```python
from build123d import *

# Parameters (mm, degrees)
F1_DEPTH       = 2.54
F3_D           = 4.4
F3_DEPTH       = 37.1856
F3_CSINK_D     = 8.96
F3_CSINK_ANGLE = 90
F3_TIP         = 1.3218933619
F4_W           = 26.1344808769
F4_H           = 86.36
F5_DEPTH       = 1.27
F7_DEPTH       = 25.4


with BuildPart() as f1:
    # F0 (on Right) → F1 (new body)
    with BuildSketch(Plane.YZ):
        Polygon((62.865, 0), (-62.865, 0), (-60.325, -86.36), (60.325, -86.36), align=None)
        Polygon((-60.325, -86.36), (-62.865, 0), (-62.865, -86.36), align=None)
        Polygon((62.865, -86.36), (62.865, 0), (60.325, -86.36), align=None)
    extrude(amount=F1_DEPTH)

    # F3
    with Locations(Plane(origin=(0, 0, 0), x_dir=(0, -1, 0), z_dir=(-1, 0, 0))):
        with Locations((-59.055, -5.08), (0, -5.08), (59.055, -5.08)):
            CounterSinkHole(F3_D / 2, F3_CSINK_D / 2, depth=F3_DEPTH, counter_sink_angle=F3_CSINK_ANGLE)
            with Locations((0, 0, -(F3_DEPTH + F3_TIP / 2))):  # 118° drill point
                Cone(0, F3_D / 2, F3_TIP, mode=Mode.SUBTRACT)

    # F4 (on face) → F5 (cut)
    with BuildSketch(Plane(origin=(0, 0, 0), x_dir=(0, -1, 0), z_dir=(-1, 0, 0))):
        with Locations((-65.7722404385, -43.18)):
            Rectangle(F4_W, F4_H)
        with Locations((65.7722404385, -43.18)):
            Rectangle(F4_W, F4_H)
    extrude(amount=-F5_DEPTH, mode=Mode.SUBTRACT)

    # F6 (on face) → F7 (cut)
    with BuildSketch(Plane(origin=(0, 0, 0), x_dir=(0, -1, 0), z_dir=(-1, 0, 0))):
        Polygon((0, -80.01), (-38.1, -86.36), (38.1, -86.36), align=None)
        Polygon((-40.64, -16.929261314), (-46.99, -16.929261314), (-50.165, -22.4285226281), (-46.99, -27.9277839421), (-40.64, -27.9277839421), (-37.465, -22.4285226281), align=None)
        Polygon((-40.64, -30.4677839421), (-46.99, -30.4677839421), (-50.165, -35.9670452561), (-46.99, -41.4663065701), (-40.64, -41.4663065701), (-37.465, -35.9670452561), align=None)
        Polygon((-40.64, -44.0063065701), (-46.99, -44.0063065701), (-50.165, -49.5055678841), (-46.99, -55.0048291981), (-40.64, -55.0048291981), (-39.0525, -52.2551985411), (-37.465, -49.5055678841), align=None)
        Polygon((-34.925, -37.2370452561), (-38.1, -42.7363065701), (-34.925, -48.2355678841), (-28.575, -48.2355678841), (-25.4, -42.7363065701), (-28.575, -37.2370452561), align=None)
        Polygon((-34.925, -34.6970452561), (-28.575, -34.6970452561), (-25.4, -29.1977839421), (-28.575, -23.698522628), (-34.925, -23.698522628), (-38.1, -29.1977839421), align=None)
        Polygon((-34.925, -21.1585226281), (-28.575, -21.1585226281), (-25.4, -15.659261314), (-28.575, -10.16), (-34.925, -10.16), (-38.1, -15.659261314), align=None)
        Polygon((-28.575, -50.7755678841), (-34.925, -50.7755678841), (-38.1, -56.2748291981), (-34.925, -61.7740905122), (-28.575, -61.7740905122), (-25.4, -56.2748291981), align=None)
        Polygon((-12.7, -29.1977839421), (-9.525, -34.6970452561), (-3.175, -34.6970452561), (0, -29.1977839421), (-3.175, -23.698522628), (-9.525, -23.698522628), align=None)
        Polygon((-12.065, -35.9670452561), (-15.24, -30.4677839421), (-21.59, -30.4677839421), (-24.765, -35.9670452561), (-21.59, -41.4663065701), (-15.24, -41.4663065701), align=None)
        Polygon((-3.175, -61.7740905122), (0, -56.2748291981), (-3.175, -50.7755678841), (-9.525, -50.7755678841), (-12.7, -56.2748291981), (-9.525, -61.7740905122), align=None)
        Polygon((-9.525, -10.16), (-12.7, -15.659261314), (-9.525, -21.1585226281), (-3.175, -21.1585226281), (0, -15.659261314), (-3.175, -10.16), align=None)
        Polygon((-12.065, -49.5055678841), (-15.24, -44.0063065701), (-21.59, -44.0063065701), (-24.765, -49.5055678841), (-21.59, -55.0048291981), (-15.24, -55.0048291981), (-13.6525, -52.2551985411), align=None)
        Polygon((-15.24, -27.9277839421), (-12.065, -22.4285226281), (-15.24, -16.929261314), (-21.59, -16.929261314), (-24.765, -22.4285226281), (-21.59, -27.9277839421), align=None)
        Polygon((-12.7, -42.7363065701), (-9.525, -48.2355678841), (-3.175, -48.2355678841), (0, -42.7363065701), (-3.175, -37.2370452561), (-9.525, -37.2370452561), align=None)
        Polygon((12.7, -29.1977839421), (15.875, -34.6970452561), (22.225, -34.6970452561), (25.4, -29.1977839421), (22.225, -23.698522628), (15.875, -23.698522628), align=None)
        Polygon((13.335, -35.9670452561), (10.16, -30.4677839421), (3.81, -30.4677839421), (0.635, -35.9670452561), (3.81, -41.4663065701), (10.16, -41.4663065701), align=None)
        Polygon((22.225, -61.7740905122), (25.4, -56.2748291981), (22.225, -50.7755678841), (15.875, -50.7755678841), (12.7, -56.2748291981), (15.875, -61.7740905122), align=None)
        Polygon((15.875, -10.16), (12.7, -15.659261314), (15.875, -21.1585226281), (22.225, -21.1585226281), (25.4, -15.659261314), (22.225, -10.16), align=None)
        Polygon((13.335, -49.5055678841), (10.16, -44.0063065701), (3.81, -44.0063065701), (0.635, -49.5055678841), (3.81, -55.0048291981), (10.16, -55.0048291981), (11.7475, -52.2551985411), align=None)
        Polygon((10.16, -27.9277839421), (13.335, -22.4285226281), (10.16, -16.929261314), (3.81, -16.929261314), (0.635, -22.4285226281), (3.81, -27.9277839421), align=None)
        Polygon((12.7, -42.7363065701), (15.875, -48.2355678841), (22.225, -48.2355678841), (25.4, -42.7363065701), (22.225, -37.2370452561), (15.875, -37.2370452561), align=None)
        Polygon((38.1, -29.1977839421), (41.275, -34.6970452561), (47.625, -34.6970452561), (50.8, -29.1977839421), (47.625, -23.698522628), (41.275, -23.698522628), align=None)
        Polygon((38.735, -35.9670452561), (35.56, -30.4677839421), (29.21, -30.4677839421), (26.035, -35.9670452561), (29.21, -41.4663065701), (35.56, -41.4663065701), align=None)
        Polygon((47.625, -61.7740905122), (50.8, -56.2748291981), (47.625, -50.7755678841), (41.275, -50.7755678841), (38.1, -56.2748291981), (41.275, -61.7740905122), align=None)
        Polygon((41.275, -10.16), (38.1, -15.659261314), (41.275, -21.1585226281), (47.625, -21.1585226281), (50.8, -15.659261314), (47.625, -10.16), align=None)
        Polygon((38.735, -49.5055678841), (35.56, -44.0063065701), (29.21, -44.0063065701), (26.035, -49.5055678841), (29.21, -55.0048291981), (35.56, -55.0048291981), (37.1475, -52.2551985411), align=None)
        Polygon((35.56, -27.9277839421), (38.735, -22.4285226281), (35.56, -16.929261314), (29.21, -16.929261314), (26.035, -22.4285226281), (29.21, -27.9277839421), align=None)
        Polygon((38.1, -42.7363065701), (41.275, -48.2355678841), (47.625, -48.2355678841), (50.8, -42.7363065701), (47.625, -37.2370452561), (41.275, -37.2370452561), align=None)
    extrude(amount=-F7_DEPTH, mode=Mode.SUBTRACT)


solid = f1.part
```
The listing builds one solid part. Answer for the finished solid, in the listing's coordinates (mm). A direction names the side the tool comes from. Coordinates: 2 decimals unless noted, no trailing zeros. Write each loop counter-clockwise with the first axis right and the second up, starting at its lowest first coordinate (ties: lowest second). Pieces come first, ordered by that corner, then holes. Notation, with made-up numbers: (-28, 52) - (27, 52) arc R24 ccw to (27, 64) - close; hole circle Ø4 at (87.5, 76). An arc over 180 degrees is marked (long way). One line per item, written item: value.
1) Find section A-A (z = -5.08). Give the vertices of the cut face in (x, y) (3 decimals).
Geometry check:
outline: (0, -52.705) - (1.27, -52.705) - (1.27, -55.845) - (2.28, -56.855) - (2.54, -56.855) - (2.54, -2.2) - (2.28, -2.2) - (0, -4.48) - close; (0, 4.48) - (2.28, 2.2) - (2.54, 2.2) - (2.54, 56.855) - (2.28, 56.855) - (1.27, 55.845) - (1.27, 52.705) - (0, 52.705) - close; (1.27, -62.865) - (2.54, -62.865) - (2.54, -61.255) - (2.28, -61.255) - (1.27, -62.265) - close; (1.27, 62.265) - (2.28, 61.255) - (2.54, 61.255) - (2.54, 62.865) - (1.27, 62.865) - close
2) Consider line 1 along Y through (x, z) = (2.5, -5.08) (3 decimals); line 2 along Z through (x, y) = (1.85, -42); line 3 along Y through (x, z) = (2.1, -28) (3 decimals). Determine where each line is inside the solid, lowest interval first. Write a range as from..to.
Geometry check:
line 1: y = -62.865..-61.255, -56.855..-2.2, 2.2..56.855, 61.255..62.865
line 2: z = -86.36..-61.77, -50.78..-48.24, -37.24..-34.7, -23.7..-21.16, -10.16..0
line 3: y = -62.865..-50.108, -38.792..-24.708, -13.392..0.692, 12.008..26.092, 37.408..62.865
3) Find section D-D (x = 0.5). Count the separate pieces of the cut face and the enclosed holes in it, and give its area (3 significant figures).
Geometry check:
separate pieces: 1
enclosed holes: 29
area: 5,880 mm2
4) A tool of negligible diameter and unlimited length cuts with its end or side. For faces 1 (the flat face through (1.25, -19.32, -83.23)), 2 (the flat face through (1, -32, -41.466)), 3 (the conical face through (2.169, -0.501, -7.336)), from which of +Z, -Z, +X, -X, +Y, -Y can it reach the whole face along a straight path? Write none if from no direction.
Geometry check:
face 1: -Z, +X, -X
face 2: +X, -X
face 3: -X
5) Find section C-C (z = -59.5). Give the vertices of the cut face in (x, y) (3 decimals).
Geometry check:
outline: (0, -52.705) - (1.27, -52.705) - (1.27, -62.865) - (2.54, -62.865) - (2.54, -48.938) - (0, -48.938) - close; (0, -39.962) - (2.54, -39.962) - (2.54, -23.538) - (0, -23.538) - close; (0, -14.562) - (2.54, -14.562) - (2.54, 1.862) - (0, 1.862) - close; (0, 10.838) - (2.54, 10.838) - (2.54, 27.262) - (0, 27.262) - close; (0, 36.238) - (2.54, 36.238) - (2.54, 62.865) - (1.27, 62.865) - (1.27, 52.705) - (0, 52.705) - close
6) Find section B-B (y = 20). Give the vertices of the cut face in (x, z), and give its area (3 significant figures).
Geometry check:
outline: (0, -83.34) - (2.54, -83.34) - (2.54, -55) - (0, -55) - close; (0, -44.01) - (2.54, -44.01) - (2.54, -41.47) - (0, -41.47) - close; (0, -30.47) - (2.54, -30.47) - (2.54, -27.93) - (0, -27.93) - close; (0, -16.93) - (2.54, -16.93) - (2.54, 0) - (0, 0) - close
area: 128 mm2
7) For a pull along Z with two mould halves and no side action, classify faces 4 (the flat face through (1.252, 13.63, -46.794)), 5 (the flat face through (2, 48, -86.36)), 6 (the flat face through (1.252, -23.79, -45.524)) as pulls with the +Z half, pulls with the -Z half, needs draft (parallel to the pull), parting line crosses it, or undercut.
Geometry check:
face 4: undercut
face 5: pulls with the -Z half
face 6: undercut
8) Each of these flat-tipped pins is pushed along its axis until it touches: pin 1 Ø5 at (y, z) = (18, -24.5) entering from +X; pin 2 Ø1.3 at (x, y) = (2, 32) entering from -Z; pin 3 Ø1 at (x, z) = (0.5, -72) entering from -Y (3 decimals); pin 4 Ø1.3 at (x, y) = (1.5, -7) entering from -Z (3 decimals). Where does it stop, or does it pass through?
Geometry check:
pin 1: passes through
pin 2: stops at z = -85.45
pin 3: stops at y = -52.705
pin 4: stops at z = -81.285
